Design review of the part built by this model. Coordinates are the model's own, in mm. Round coordinates to 2 decimals unless told otherwise and drop trailing zeros. Order: outer loops, then holes, each group sorted by start corner. A loop starts at its lowest first (then second) coordinate and runs counter-clockwise, first axis right, second up. Notation, with made-up numbers: (-30, -33.75) - (18, -33.75) arc R13 cw to (18, -12.75) - close; hole circle Ø1 at (4.25, 64.5). An arc over 180 degrees is marked (long way). Use CSV: the item, a comma, the result in double quotes.
from build123d import *

# Parameters (mm, degrees)
BOSS_EXTRUDE1_DEPTH = 5


with BuildPart() as part:
    # Sketch1 → Boss-Extrude1 (new body)
    with BuildSketch(Plane.XY):
        Polygon((305.05, 56), (349.05, 56), (349.05, 61), (393.05, 61), (393.05, 56), (447, 56), (447, 0), (444.06, 0), (444.06, 4), (435.06, 4), (435.06, 0), (434, 0), (434, -5), (396, -5), (396, 0), (352, 0), (352, -5), (308, -5), (308, 0), (264, 0), (264, -5), (220, -5), (220, 0), (176, 0), (176, -5), (132, -5), (132, 0), (88, 0), (88, -5), (44, -5), (44, 0), (0, 0), (-7, 0), (-7, 56), (-2.95, 56), (-2.95, 61), (41.05, 61), (41.05, 56), (85.05, 56), (85.05, 61), (129.05, 61), (129.05, 56), (173.05, 56), (173.05, 61), (217.05, 61), (217.05, 56), (261.05, 56), (261.05, 61), (305.05, 61), align=None)
    extrude(amount=BOSS_EXTRUDE1_DEPTH)


solid = part.part
1) We need section A-A (x = 192). Give the boundary of the cut face in (y, z).
Data:
outline,"(0, 0) - (61, 0) - (61, 5) - (0, 5) - close"
2) Insertion check: pin 1 Ø1.5 at (y, z) = (-2, 3.5) entering from -X; pin 2 Ø2.5 at (x, z) = (412, 2.5) entering from +Y; pin 3 Ø2.5 at (y, z) = (57.5, 1.5) entering from -X. Each pin has a flat end and moves straight along its axis. Give the tip position at first contact, or say it passes through.
Data:
pin 1,"stops at x = 44"
pin 2,"stops at y = 56"
pin 3,"stops at x = -2.95"
3) To check wall thickness, follow L1, parallel to X at y = 57, z = 1; L2, parallel to Y at x = 376.5, z = 3.1; L3, parallel to Y at x = 428, z = 1.9. State the ranges of each line that lie inside material, in increasing order. Write a range as from..to.
Data:
L1,"x = -2.95..41.05, 85.05..129.05, 173.05..217.05, 261.05..305.05, 349.05..393.05"
L2,"y = 0..61"
L3,"y = -5..56"
